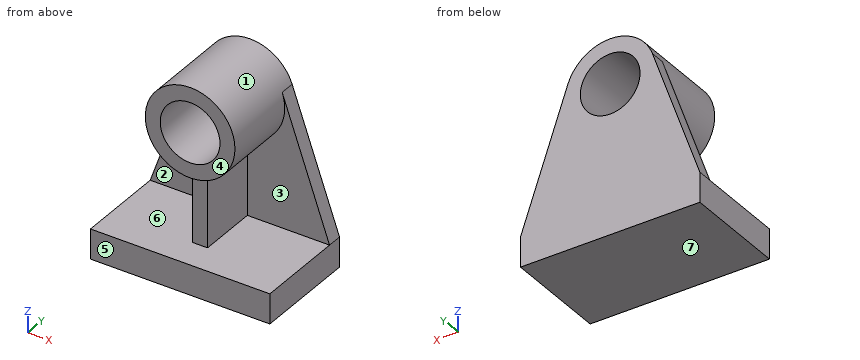
from build123d import *

# Parameters (mm, degrees)
F2_DEPTH  = 25.4
F3_W      = 304.8
F3_H      = 50.8
F4_DEPTH  = 152.4
F5_W      = 25.4
F5_H      = 203.2
F6_DEPTH  = 101.6
F7_R      = 76.2
F8_DEPTH  = 127
F9_R      = 50.8
F10_DEPTH = 152.401


# Not quite as in the source:
# - a variable given as a bare number and used for a length is read in inches; the dataset says mm whatever the document's units were


with BuildPart() as f2:
    # F1 (on Front) → F2 (new body)
    with BuildSketch(Plane.XZ):
        with BuildLine():
            Line((-304.8, 0), (0, 0))
            Line((0, 0), (0, 50.8))
            Line((0, 50.8), (-80.5318662816, 279.3261002888))
            ThreePointArc((-80.5318662816, 279.3261002888), (-152.4, 330.2), (-224.2681337184, 279.3261002888))
            Line((-224.2681337184, 279.3261002888), (-304.8, 50.8))
            Line((-304.8, 50.8), (-304.8, 0))
        make_face()
    extrude(amount=F2_DEPTH)

    # F3 (on face) → F4 (join)
    with BuildSketch(Plane.XZ.offset(25.4)):
        with Locations((-152.4, 25.4)):
            Rectangle(F3_W, F3_H)
    extrude(amount=F4_DEPTH)

    # F5 (on face) → F6 (join)
    with BuildSketch(Plane.XZ.offset(25.4)):
        with Locations((-152.4, 152.4)):
            Rectangle(F5_W, F5_H)
    extrude(amount=F6_DEPTH)

    # F7 (on face) → F8 (join)
    with BuildSketch(Plane.XZ.offset(25.4)):
        with Locations((-152.4, 254)):
            Circle(F7_R)
    extrude(amount=F8_DEPTH)

    # F9 (on face) → F10 (cut, through all)
    with BuildSketch(Plane.XZ.offset(152.4)):
        with Locations((-152.4, 254)):
            Circle(F9_R)
    extrude(amount=-F10_DEPTH, mode=Mode.SUBTRACT)


solid = f2.part
The listing builds one solid part. Answer for the finished solid, in the listing's coordinates (mm). Face numbers are marked on the shaded views. A direction names the side the tool comes from. Round coordinates to 2 decimals unless told otherwise and drop trailing zeros. Write each loop counter-clockwise with the first axis right and the second up, starting at its lowest first coordinate (ties: lowest second). Pieces come first, ordered by that corner, then holes. Notation, with made-up numbers: (57, 89) - (84, 89) arc R19 ccw to (84, 117) - close; hole circle Ø6 at (-22.75, -23.75). An arc over 180 degrees is marked (long way). Use one line per item in the form item = value. Start each with the question number.
Item 1: A cutting plane is placed at A-A (y = -45). Write down the section's boundary in (x, z).
Item 2: A cutting plane is placed at D-D (z = 254). Write down the section's boundary in (x, y).
Item 3: Flat-ended cylindrical pins translate along their axes: pin 1 Ø12 at (x, y) = (-190, -135) entering from +Z; pin 2 Ø3 at (y, z) = (-29, 197) entering from +X; pin 3 Ø5 at (y, z) = (-80.5, 287) entering from -X. Find the tip coordinate at first contact, or state that the pin passes through.
Item 4: Determine the mould class of the marked faces 5, 6 and 7 for opening direction Z: +Z half, -Z half, draft (parallel to the pull), parting line (faces both ways), or undercut.
Item 5: A cutting plane is placed at C-C (y = -131.5). Write down the section's boundary in (x, z).
Item 6: A cutting plane is placed at B-B (x = -152.4). Write down the section's boundary in (y, z).
Item 7: Find the intervals of material crossed by line 1 (Z direction, x = -152.4, y = -48.5); line 2 (Z direction, x = -109.5, y = -47); line 3 (Z direction, x = -167.5, y = -152), in increasing order. Write a range as [from, to].
Item 8: A tool of negligible diameter and unlimited length cuts with its end or side. For the marked faces 1, 2, 3 and 4, from which of +Z, -Z, +X, -X, +Y, -Y can it reach the whole face along a straight path? Write none if from no direction.
The answers:
q1.outline = (-304.8, 0) - (0, 0) - (0, 50.8) - (-139.7, 50.8) - (-139.7, 178.87) arc R76.2 ccw (long way) to (-165.1, 178.87) - (-165.1, 50.8) - (-304.8, 50.8) - close; hole circle Ø101.6 at (-152.4, 254)
q2.outline = (-233.19, -25.4) - (-228.6, -25.4) - (-228.6, -152.4) - (-203.2, -152.4) - (-203.2, 0) - (-233.19, 0) - close; (-101.6, -152.4) - (-76.2, -152.4) - (-76.2, -25.4) - (-71.61, -25.4) - (-71.61, 0) - (-101.6, 0) - close
q3.pin_1 = 323.34
q3.pin_2 = -100.19
q3.pin_3 = -222.23
q4.face_5 = draft
q4.face_6 = undercut
q4.face_7 = -Z half
q5.outline = (-304.8, 0) - (0, 0) - (0, 50.8) - (-304.8, 50.8) - close; circle Ø152.4 at (-152.4, 254); hole circle Ø101.6 at (-152.4, 254)
q6.outline = (-177.8, 0) - (0, 0) - (0, 203.2) - (-152.4, 203.2) - (-152.4, 177.8) - (-127, 177.8) - (-127, 50.8) - (-177.8, 50.8) - close; (-152.4, 304.8) - (0, 304.8) - (0, 330.2) - (-152.4, 330.2) - close
q7.line_1 = [0, 203.2], [304.8, 330.2]
q7.line_2 = [0, 50.8], [191.02, 226.79], [281.21, 316.98]
q7.line_3 = [0, 50.8], [179.31, 205.5], [302.5, 328.69]
q8.face_1 = -Y
q8.face_2 = -X, -Y
q8.face_3 = +X, -Y
q8.face_4 = +Z, +X, -X, -Y
